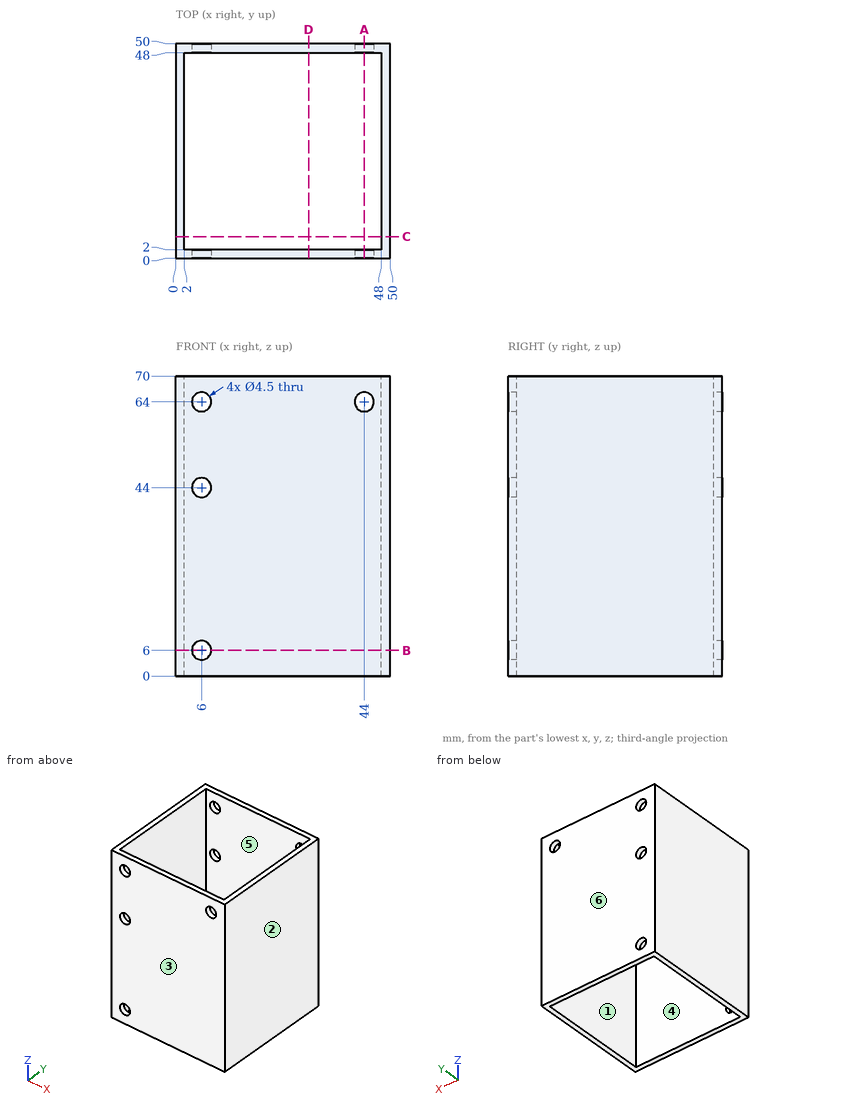
The drawing under review shows one solid part. Ordinate dimensions are in mm from its lowest x, y, z. A direction names the side the tool comes from. Give positions to 0.01 mm unless a question says otherwise; leave off trailing zeros. Order: outer loops, then holes, each group sorted by start corner. A loop starts at its lowest first (then second) coordinate and runs counter-clockwise, first axis right, second up. Notation, with made-up numbers: (23.5, -0.75) -> (73.5, -0.75) arc R22 cw to (73.5, 25.25) -> close; hole circle Ø2 at (65.25, 23.5). An arc over 180 degrees is marked (long way). Write item = value, one per line. Start each with the question number.
(1) For pin 1 (5 mm diameter, centred on x = 6, z = 64, fed in from +Y); pin 2 (3.5 mm diameter, centred on x = 44, z = 64, fed in from -Y), all flat-tipped, find the tip position at first contact; note any pin that passes through.
(2) Mouldability with a two-part tool opening along X and no side actions: class the marked faces 1, 2, 3 and 4 as +X half, -X half, draft (parallel to the pull), parting line (faces both ways), or undercut.
(3) We need section B-B on z = 6. Write out the cut boundary in (x, y).
(4) To check wall thickness, follow line 1 along X through (y, z) = (49, 64); line 2 along Z through (x, y) = (6, 48.8); line 3 along Z through (x, y) = (44, 0.95). State the ranges of each line that lie inside material, in increasing order.
(5) For the marked faces 5 and 6, list the 3-axis set-ups (+Z, -Z, +X, -X, +Y, -Y) from which the entire face can be reached by the end or side of a thin tool; tool diameter is ignored.
(6) We need section A-A on x = 44. Write out the cut boundary in (y, z).
(7) We need section C-C on y = 5. Write out the cut boundary in (x, z).
Numbers:
q1.pin_1 = 50
q1.pin_2 = through
q2.face_1 = undercut
q2.face_2 = +X half
q2.face_3 = draft
q2.face_4 = undercut
q3.outline = (0, 0) -> (3.75, 0) -> (3.75, 2) -> (2, 2) -> (2, 48) -> (3.75, 48) -> (3.75, 50) -> (0, 50) -> close; (8.25, 0) -> (50, 0) -> (50, 50) -> (8.25, 50) -> (8.25, 48) -> (48, 48) -> (48, 2) -> (8.25, 2) -> close
q4.line_1 = 0 to 3.75, 8.25 to 41.75, 46.25 to 50
q4.line_2 = 0 to 3.75, 8.25 to 41.75, 46.25 to 61.75, 66.25 to 70
q4.line_3 = 0 to 61.75, 66.25 to 70
q5.face_5 = +Z, -Z
q5.face_6 = +Z, -Z, +X, -X, +Y
q6.outline = (0, 0) -> (2, 0) -> (2, 61.75) -> (0, 61.75) -> close; (0, 66.25) -> (2, 66.25) -> (2, 70) -> (0, 70) -> close; (48, 0) -> (50, 0) -> (50, 61.75) -> (48, 61.75) -> close; (48, 66.25) -> (50, 66.25) -> (50, 70) -> (48, 70) -> close
q7.outline = (0, 0) -> (2, 0) -> (2, 70) -> (0, 70) -> close; (48, 0) -> (50, 0) -> (50, 70) -> (48, 70) -> close
